The figure shows three views and two pictorial views of one solid part (mm, origin at its lowest corner). Answer the questions. Coordinates: 2 decimals unless noted, no trailing zeros. Order: outer loops, then holes, each group sorted by start corner. A loop starts at its lowest first (then second) coordinate and runs counter-clockwise, first axis right, second up. Notation, with made-up numbers: (-19.75, 72) -> (15.25, 72) arc R7 cw to (15.25, 84) -> close; hole circle Ø2 at (-17, -4.5). An arc over 180 degrees is marked (long way). Write item = value, one per line. Start each with the question number.
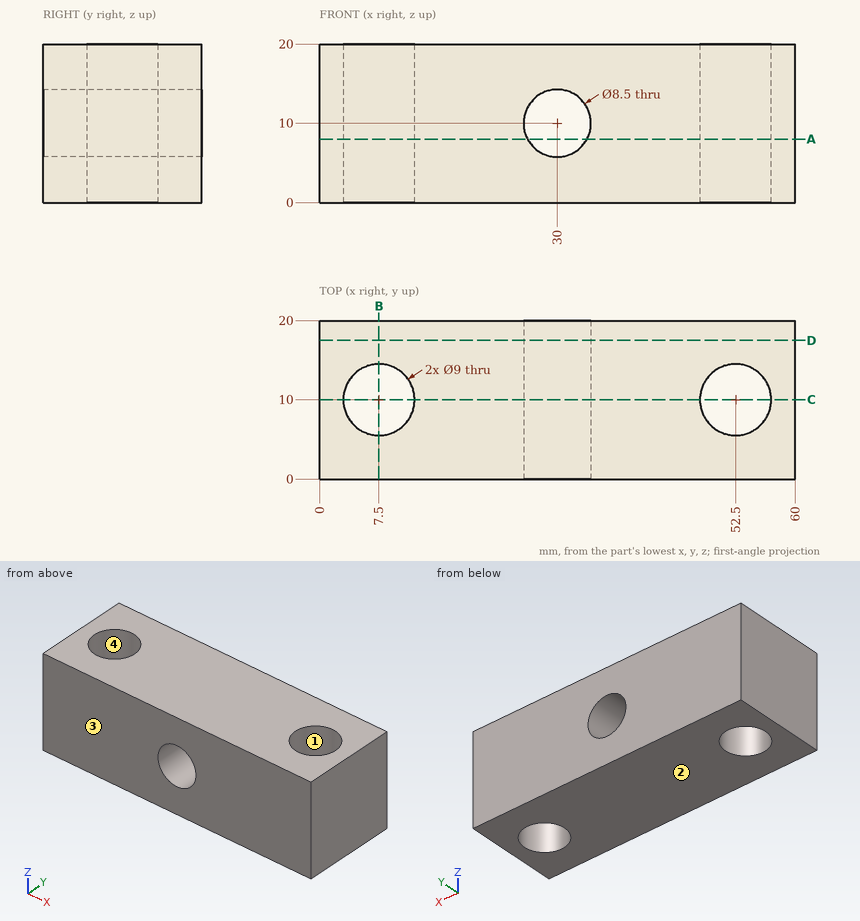
Item 1: Section A-A, the plane z = 8 is taken. Give the vertices of the cut face in (x, y), then the cut area to 3 significant figures.
Item 2: Each of these flat-tipped pins is pushed along its axis until it touches: pin 1 (1 mm diameter, centred on x = 12.5, y = 17, fed in from -Z); pin 2 (7 mm diameter, centred on x = 7.5, y = 10, fed in from +Z). Where does it stop, or does it pass through?
Item 3: Consider probe 1 along Y at (x, z) = (7.5, 7.5); probe 2 along X at (y, z) = (11, 10); probe 3 along X at (y, z) = (11.25, 8.75). Determine where each line is inside the solid, lowest interval first.
Item 4: For a pull along Y with two mould halves and no side action, classify the marked faces 1, 2, 3 and 4 as pulls with the +Y half, pulls with the -Y half, needs draft (parallel to the pull), parting line crosses it, or undercut.
Item 5: Section C-C, the plane y = 10 is taken. Give the vertices of the cut face in (x, z).
Item 6: Section B-B, the plane x = 7.5 is taken. Give the vertices of the cut face in (y, z).
Item 7: Section D-D, the plane y = 17.5 is taken. Give the vertices of the cut face in (x, z), then the cut area to 3 significant figures.
A:
q1.outline = (0, 0) -> (26.25, 0) -> (26.25, 20) -> (0, 20) -> close; (33.75, 0) -> (60, 0) -> (60, 20) -> (33.75, 20) -> close; hole circle Ø9 at (7.5, 10); hole circle Ø9 at (52.5, 10)
q1.area = 923 mm^2
q2.pin_1 = 0
q2.pin_2 = through
q3.probe_1 = 0 to 5.5, 14.5 to 20
q3.probe_2 = 0 to 3.11, 11.89 to 25.75, 34.25 to 48.11, 56.89 to 60
q3.probe_3 = 0 to 3.18, 11.82 to 25.94, 34.06 to 48.18, 56.82 to 60
q4.face_1 = undercut
q4.face_2 = needs draft
q4.face_3 = pulls with the -Y half
q4.face_4 = undercut
q5.outline = (0, 0) -> (3, 0) -> (3, 20) -> (0, 20) -> close; (12, 0) -> (48, 0) -> (48, 20) -> (12, 20) -> close; (57, 0) -> (60, 0) -> (60, 20) -> (57, 20) -> close; hole circle Ø8.5 at (30, 10)
q6.outline = (0, 0) -> (5.5, 0) -> (5.5, 20) -> (0, 20) -> close; (14.5, 0) -> (20, 0) -> (20, 20) -> (14.5, 20) -> close
q7.outline = (0, 0) -> (60, 0) -> (60, 20) -> (0, 20) -> close; hole circle Ø8.5 at (30, 10)
q7.area = 1,140 mm^2
